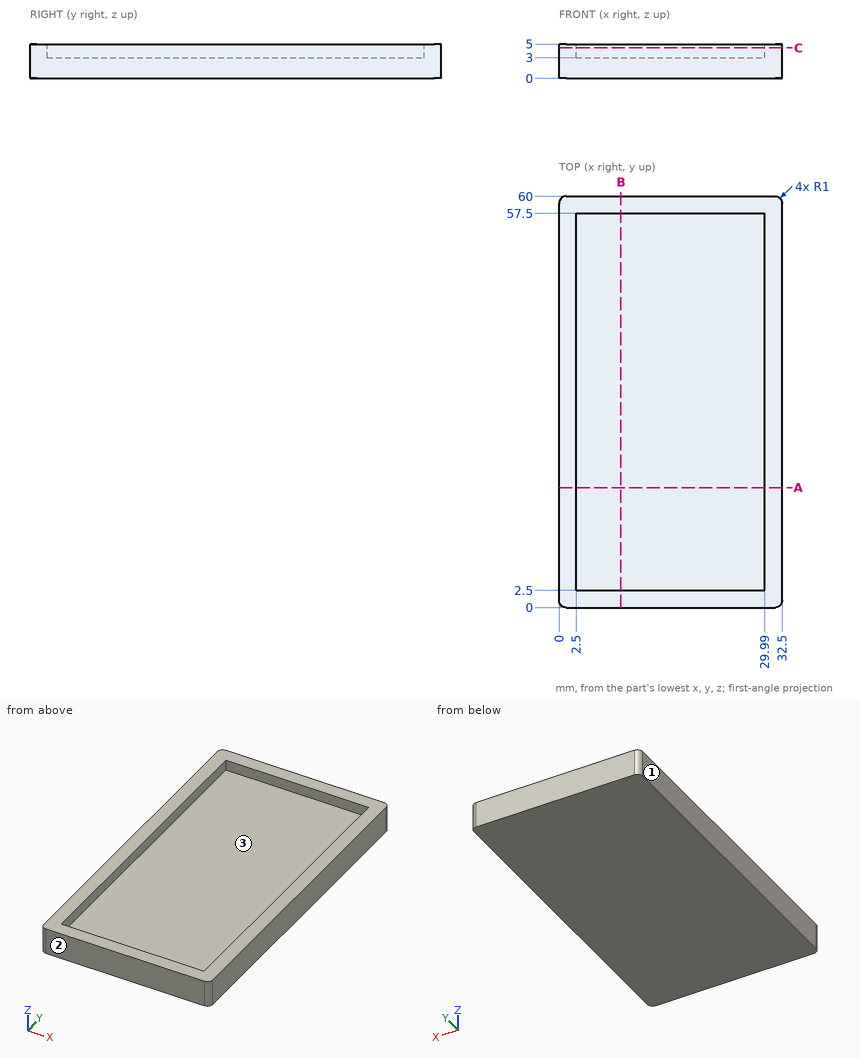
Can you work these out from the drawing? Everything is in mm from the part's minimum corner. Coordinates: 2 decimals unless noted, no trailing zeros. Loops run counter-clockwise (first coordinate to the right, second up) from the corner with the lowest first, then second, coordinate; pieces in that order, holes last. Notation, with made-up numbers: M 63,14 L 116,14 A21 ccw 116,36 Z; hole C 48.5,-33.5 d7. An arc over 180 degrees is marked long. Put each result on its own line as item: value. Start each with the question number.
(1) Suppose I cut it at A-A on y = 17.5. Please give me the cut outline in (x, z), then the cut area to 3 significant figures.
(2) Thinking about a two-plate mould opening in Y: for the marked faces 1, 2 and 3, which applies, pulls with the +Y half, pulls with the -Y half, needs draft (parallel to the pull), parting line crosses it, or undercut?
(3) Suppose I cut it at C-C on z = 4.45. Please give me the cut outline in (x, y), then the cut area to 3 significant figures.
(4) I need wall thicknesses on line 1 (X direction, y = 39, z = 4.15); line 2 (Y direction, x = 21.5, z = 4.3); line 3 (Z direction, x = 13.5, y = 23). Which ranges of each line are inside material? Lowest first, please. Write a range as from..to.
(5) Will this pin go through, and if not, where does the flat tip stop? P1, Ø13.5, axis at x = 22, y = 36.5, coming from the +Z side.
(6) Suppose I cut it at B-B on x = 9. Please give me the cut outline in (y, z), then the cut area to 3 significant figures.
Solutions:
1. outline: M 0,0 L 32.5,0 L 32.5,5 L 29.99,5 L 29.99,3 L 2.5,3 L 2.5,5 L 0,5 Z
1. area: 108 mm2
2. face 1: needs draft
2. face 2: pulls with the -Y half
2. face 3: undercut
3. outline: M 0,1 A1 ccw 1,0 L 31.5,0 A1 ccw 32.5,1 L 32.5,59 A1 ccw 31.5,60 L 1,60 A1 ccw 0,59 Z; hole M 2.5,2.5 L 29.99,2.5 L 29.99,57.5 L 2.5,57.5 Z
3. area: 437 mm2
4. line 1: x = 0..2.5, 29.99..32.5
4. line 2: y = 0..2.5, 57.5..60
4. line 3: z = 0..3
5. P1: stops at z = 3
6. outline: M 0,0 L 60,0 L 60,5 L 57.5,5 L 57.5,3 L 2.5,3 L 2.5,5 L 0,5 Z
6. area: 190 mm2
